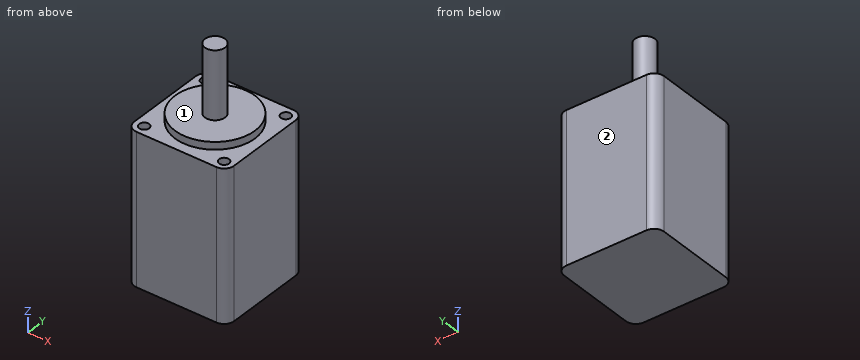
```python
from build123d import *

# Parameters (mm, degrees)
SKETCH1_W           = 20
SKETCH1_H           = 20
BOSS_EXTRUDE1_DEPTH = 30
SKETCH2_R           = 1
CUT_EXTRUDE1_DEPTH  = 6
FILLET1_R           = 2
SKETCH3_R           = 8
BOSS_EXTRUDE2_DEPTH = 1.5
SKETCH4_R           = 2
BOSS_EXTRUDE3_DEPTH = 13.5


with BuildPart() as part:
    # Sketch1 → Boss-Extrude1 (new body)
    with BuildSketch(Plane.XY):
        Rectangle(SKETCH1_W, SKETCH1_H)
    extrude(amount=-BOSS_EXTRUDE1_DEPTH)

    # Sketch2 → Cut-Extrude1 (cut)
    with BuildSketch(Plane.XY):
        with Locations((-8, 8)):
            Circle(SKETCH2_R)
        with Locations((8, 8)):
            Circle(SKETCH2_R)
        with Locations((8, -8)):
            Circle(SKETCH2_R)
        with Locations((-8, -8)):
            Circle(SKETCH2_R)
    extrude(amount=-CUT_EXTRUDE1_DEPTH, mode=Mode.SUBTRACT)

    # Fillet1
    fillet1_edges = [part.edges().sort_by_distance(p)[0] for p in [
        (10, -10, -15),
        (-10, -10, -15),
        (-10, 10, -15),
        (10, 10, -15),
    ]]
    fillet(fillet1_edges, radius=FILLET1_R)

    # Sketch3 → Boss-Extrude2 (add)
    with BuildSketch(Plane.XY):
        Circle(SKETCH3_R)
    extrude(amount=BOSS_EXTRUDE2_DEPTH)

    # Sketch4 → Boss-Extrude3 (add)
    with BuildSketch(Plane.XY.offset(1.5)):
        Circle(SKETCH4_R)
    extrude(amount=BOSS_EXTRUDE3_DEPTH)


solid = part.part
```
Input: part model. Units: mm. Frame: model coordinates. Face numbers are marked on the shaded views. A direction names the side the tool comes from. Coordinates: 2 decimals unless noted, no trailing zeros. Loops run counter-clockwise (first coordinate to the right, second up) from the corner with the lowest first, then second, coordinate; pieces in that order, holes last.
Q1. Contact query for flat-ended pins moving along their axis: pin 1 (1 mm diameter, centred on x = -8, y = -8, fed in from +Z); pin 2 (2 mm diameter, centred on x = 8.5, y = -7.5, fed in from +Z); pin 3 (6 mm diameter, centred on x = 4, y = 7.5, fed in from +Z). Output: stop coordinate, or through.
Results are:
pin 1: stops at z = -6
pin 2: stops at z = 0
pin 3: stops at z = 1.5
Q2. Section D-D, the plane y = 0. Return the cut outline in (x, z).
Results are:
outline: (-10, -30) - (10, -30) - (10, 0) - (8, 0) - (8, 1.5) - (2, 1.5) - (2, 15) - (-2, 15) - (-2, 1.5) - (-8, 1.5) - (-8, 0) - (-10, 0) - close
Q3. Section C-C, the plane x = -4.5. Return the cut outline in (y, z).
Results are:
outline: (-10, -30) - (10, -30) - (10, 0) - (6.61, 0) - (6.61, 1.5) - (-6.61, 1.5) - (-6.61, 0) - (-10, 0) - close
Q4. Line query: line 1 along Y through (x, z) = (8, -1.45); line 2 along Z through (x, y) = (-7.5, -0.75); line 3 along Z through (x, y) = (-6.25, 6.5). Output: solid intervals per line, ascending.
Results are:
line 1: y = -10 to -9, -7 to 7, 9 to 10
line 2: z = -30 to 1.5
line 3: z = -30 to 0
Q5. Set-up query: the marked faces 1 and 2. Return all of +Z, -Z, +X, -X, +Y, -Y with unobstructed straight access to the full face (end or side cutting, diameter ignored); none if empty.
Results are:
face 1: +Z
face 2: +Z, -Z, +X, -X, +Y
Q6. Section A-A, the plane z = -4. Return the cut outline in (x, y).
Results are:
outline: (-10, -8) arc R2 ccw to (-8, -10) - (8, -10) arc R2 ccw to (10, -8) - (10, 8) arc R2 ccw to (8, 10) - (-8, 10) arc R2 ccw to (-10, 8) - close; hole circle Ø2 at (-8, -8); hole circle Ø2 at (-8, 8); hole circle Ø2 at (8, -8); hole circle Ø2 at (8, 8)
Q7. Section B-B, the plane y = 7.5. Return the cut outline in (x, z), and give its area (3 significant figures).
Results are:
outline: (-10, -30) - (10, -30) - (10, 0) - (8.87, 0) - (8.87, -6) - (7.13, -6) - (7.13, 0) - (2.78, 0) - (2.78, 1.5) - (-2.78, 1.5) - (-2.78, 0) - (-7.13, 0) - (-7.13, -6) - (-8.87, -6) - (-8.87, 0) - (-10, 0) - close
area: 588 mm2
